The drawing under review shows one solid part. Ordinate dimensions are in mm from its lowest x, y, z. A direction names the side the tool comes from. Give positions to 0.01 mm unless a question says otherwise; leave off trailing zeros. Loops run counter-clockwise (first coordinate to the right, second up) from the corner with the lowest first, then second, coordinate; pieces in that order, holes last. Notation, with made-up numbers: (-22.5, 70) - (1.5, 70) arc R17 ccw to (1.5, 101) - close; hole circle Ø6 at (56, 8). An arc over 180 degrees is marked (long way). Write each question's results on one line, items separated by ' | '.
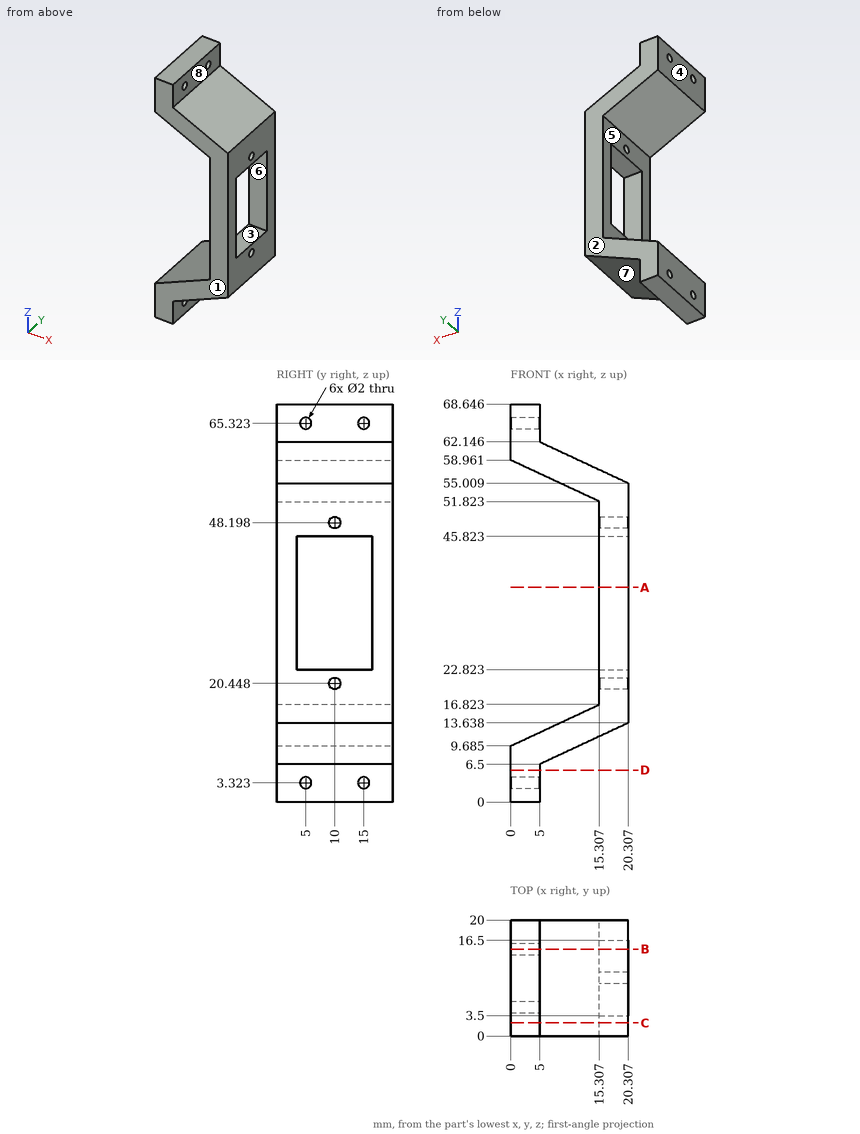
(1) Insertion check: P1, Ø1.5, axis at x = 16, y = 9.5, coming from the -Z side; P2, Ø7, axis at y = 7, z = 2.5, coming from the +X side; P3, Ø4, axis at x = 18, y = 9.5, coming from the +Z side. Each pin has a flat end and moves straight along its axis. Give the tip position at first contact, or say it passes through.
Answers below:
P1: z = 11.28 | P2: x = 5 | P3: z = 57.02
(2) Take a section at C-C on y = 2.25. Give the boundary of the cut face in (x, z) (1 decimal).
Answers below:
outline: (0, 0) - (5, 0) - (5, 6.5) - (20.3, 13.6) - (20.3, 55) - (5, 62.1) - (5, 68.6) - (0, 68.6) - (0, 59) - (15.3, 51.8) - (15.3, 16.8) - (0, 9.7) - close
(3) Wall thickness on line 1 along Z through (x, y) = (16.25, 9.5) (1 decimal); line 2 along X through (y, z) = (17.5, 43); line 3 along X through (y, z) = (10, 63.5): over which ranges is each line inside the solid? List them lowest first. Write a range as from..to.
Answers below:
line 1: 11.7..19.6, 21.3..22.8, 45.8..47.3, 49.1..56.9 | line 2: 15.31..20.31 | line 3: 0..5
(4) Draft analysis for pull direction Y (two halves, no side actions). For the marked faces 1, 2, 3 and 4, state which applies: pulls with the +Y half, pulls with the -Y half, needs draft (parallel to the pull), parting line crosses it, or undercut.
Answers below:
face 1: pulls with the -Y half | face 2: pulls with the +Y half | face 3: undercut | face 4: needs draft
(5) Take a section at A-A on z = 37. Give the boundary of the cut face in (x, y).
Answers below:
outline: (15.31, 0) - (20.31, 0) - (20.31, 3.5) - (15.31, 3.5) - close; (15.31, 16.5) - (20.31, 16.5) - (20.31, 20) - (15.31, 20) - close
(6) Tool access review of the marked faces 5, 6, 7 and 8: name each direction out of +Z, -Z, +X, -X, +Y, -Y from which nothing blocks a thin tool from reaching the whole face with its end or side.
Answers below:
face 5: -X, +Y, -Y | face 6: +X, -X | face 7: -Z, +X, +Y, -Y | face 8: +Z, +X, +Y, -Y
(7) Take a section at B-B on y = 15. Give the boundary of the cut face in (x, z) (1 decimal), plus the area to 3 significant figures.
Answers below:
outline: (0, 0) - (5, 0) - (5, 2.3) - (0, 2.3) - close; (0, 4.3) - (5, 4.3) - (5, 6.5) - (20.3, 13.6) - (20.3, 22.8) - (15.3, 22.8) - (15.3, 16.8) - (0, 9.7) - close; (0, 59) - (15.3, 51.8) - (15.3, 45.8) - (20.3, 45.8) - (20.3, 55) - (5, 62.1) - (5, 64.3) - (0, 64.3) - close; (0, 66.3) - (5, 66.3) - (5, 68.6) - (0, 68.6) - close | area: 306 mm2
(8) Take a section at D-D on z = 5.5. Give the boundary of the cut face in (x, y).
Answers below:
outline: (0, 0) - (5, 0) - (5, 20) - (0, 20) - close
